CAD build for the part. Positions are in the model's coordinates, mm. A direction names the side the tool comes from. Round coordinates to 2 decimals unless told otherwise and drop trailing zeros. Write each loop counter-clockwise with the first axis right and the second up, starting at its lowest first coordinate (ties: lowest second). Pieces come first, ordered by that corner, then holes. Notation, with made-up numbers: (51.25, 89) -> (85.25, 89) arc R21 cw to (85.25, 102) -> close; hole circle Ø8 at (72.5, 11.25). An arc over 180 degrees is marked (long way). Answer in a Markdown table with one row per item. Add a question column.
```python
from build123d import *

# Parameters (mm, degrees)
SKETCH1_R                       = 60
SKETCH1_R_2                     = 45
BOSS_EXTRUDE1_DEPTH             = 3
CUT_EXTRUDE1_DEPTH              = 85.905830189
CIRPATTERN1_COUNT               = 8
SKETCH3_R                       = 2.1
CUT_EXTRUDE2_DEPTH              = 85.905830189
CIRPATTERN2_COUNT               = 4
SCHNITT_LINEAR_AUSTRAGEN1_DEPTH = 85.905830189
VERRUNDUNG2_R                   = 2
KREISMUSTER7_COUNT              = 4
VERRUNDUNG2_OF_KREISMUSTER7_R   = 2


with BuildPart() as part:
    # Sketch1 → Boss-Extrude1 (new body)
    with BuildSketch(Plane(origin=(0, 0, 0), x_dir=(1, 0, 0), z_dir=(0, 1, 0))):
        with Locations(Location((0, 0, 0), (0, 0, 270))):
            Circle(SKETCH1_R)
        with Locations(Location((0, 0, 0), (0, 0, 270))):
            Circle(SKETCH1_R_2, mode=Mode.SUBTRACT)
    extrude(amount=BOSS_EXTRUDE1_DEPTH)

    # Sketch2 → Cut-Extrude1 (cut, through all)
    with BuildSketch(Plane(origin=(0, 3, 0), x_dir=(1, 0, 0), z_dir=(0, 1, 0))):
        with BuildLine():
            Line((12.399026137, 46.273795509), (12.153476553, 45.357391985))
            ThreePointArc((12.153476553, 45.357391985), (12.332388249, 43.876840862), (13.485952537, 42.931679261))
            Line((13.485952537, 42.931679261), (-13.485952537, 42.931679261))
            ThreePointArc((-13.485952537, 42.931679261), (-12.332388249, 43.876840862), (-12.153476553, 45.357391985))
            Line((-12.153476553, 45.357391985), (-12.399026137, 46.273795509))
            ThreePointArc((-12.399026137, 46.273795509), (-12.051156799, 48.63074892), (-10.0950767, 49.990893435))
            ThreePointArc((-10.0950767, 49.990893435), (0, 51), (10.0950767, 49.990893435))
            ThreePointArc((10.0950767, 49.990893435), (12.051156799, 48.63074892), (12.399026137, 46.273795509))
        make_face()
    cut_extrude1 = extrude(amount=-CUT_EXTRUDE1_DEPTH, mode=Mode.SUBTRACT)

    # CirPattern1: Cut-Extrude1 ×8 about axis
    cirpattern1_axis = Axis((0, 0, 0), (0, 1, 0))
    for i in range(1, CIRPATTERN1_COUNT):
        add(cut_extrude1.rotate(cirpattern1_axis, i * 360 / CIRPATTERN1_COUNT), mode=Mode.SUBTRACT)

    # Sketch3 → Cut-Extrude2 (cut, through all)
    with BuildSketch(Plane(origin=(0, 3, 0), x_dir=(1, 0, 0), z_dir=(0, 1, 0))):
        with Locations(Location((38.890872965, 38.890872965, 0), (0, 0, 270))):
            Circle(SKETCH3_R)
    cut_extrude2 = extrude(amount=-CUT_EXTRUDE2_DEPTH, mode=Mode.SUBTRACT)

    # CirPattern2: Cut-Extrude2 ×4 about axis
    cirpattern2_axis = Axis((0, 0, 0), (0, 1, 0))
    for i in range(1, CIRPATTERN2_COUNT):
        add(cut_extrude2.rotate(cirpattern2_axis, i * 360 / CIRPATTERN2_COUNT), mode=Mode.SUBTRACT)

    # Skizze1 → Schnitt-Linear austragen1 (cut, through all)
    with BuildSketch(Plane(origin=(0, 3, 0), x_dir=(1, 0, 0), z_dir=(0, 1, 0))):
        with BuildLine():
            Line((-12.986376836, 58.577760427), (-12.120618381, 54.672576399))
            ThreePointArc((-12.120618381, 54.672576399), (0, 56), (12.120618381, 54.672576399))
            Line((12.120618381, 54.672576399), (12.986376836, 58.577760427))
            ThreePointArc((12.986376836, 58.577760427), (0, 60), (-12.986376836, 58.577760427))
        make_face()
    schnitt_linear_austragen1 = extrude(amount=-SCHNITT_LINEAR_AUSTRAGEN1_DEPTH, mode=Mode.SUBTRACT)

    # Verrundung2
    verrundung2_edges = [part.edges().sort_by_distance(p)[0] for p in [
        (-12.986376836, 1.5, -58.577760427),
        (-12.120618381, 1.5, -54.672576399),
        (12.986376836, 1.5, -58.577760427),
        (12.120618381, 1.5, -54.672576399),
    ]]
    fillet(verrundung2_edges, radius=VERRUNDUNG2_R - 0.0001)  # a hair under: the kernel refuses the full size

    # Kreismuster7: Schnitt-Linear austragen1 ×4 about axis
    kreismuster7_axis = Axis((0, 0, 0), (0, 1, 0))
    for i in range(1, KREISMUSTER7_COUNT):
        add(schnitt_linear_austragen1.rotate(kreismuster7_axis, i * 360 / KREISMUSTER7_COUNT), mode=Mode.SUBTRACT)

    # Verrundung2 of Kreismuster7
    verrundung2_of_kreismuster7_edges = [part.edges().sort_by_distance(p)[0] for p in [
        (-58.577760427, 1.5, 12.986376836),
        (-54.672576399, 1.5, 12.120618381),
        (-58.577760427, 1.5, -12.986376836),
        (-54.672576399, 1.5, -12.120618381),
        (12.986376836, 1.5, 58.577760427),
        (12.120618381, 1.5, 54.672576399),
        (-12.986376836, 1.5, 58.577760427),
        (-12.120618381, 1.5, 54.672576399),
        (58.577760427, 1.5, -12.986376836),
        (54.672576399, 1.5, -12.120618381),
        (58.577760427, 1.5, 12.986376836),
        (54.672576399, 1.5, 12.120618381),
    ]]
    fillet(verrundung2_of_kreismuster7_edges, radius=VERRUNDUNG2_OF_KREISMUSTER7_R - 0.0001)  # a hair under: the kernel refuses the full size


solid = part.part
```
Item 1: Two-plate mould, pull along X, no slides. Class faces 1 (the cylindrical face through (51, 2, 0)), 2 (the flat face through (43.4, 3, -13.2)), 3 (the cylindrical face through (-56, 2, 0)): +X half, -X half, draft (parallel to the pull), parting line (faces both ways), or undercut.
Item 2: Saw through at C-C on y = 1.8. Count the separate pieces of the cut face and the enclosed holes in it, then the cut area to 3 significant figures.
Item 3: Tool access for faces 4 (the cylindrical face through (0, 2, -56)), 5 (the cylindrical face through (-17.272, 1.479, 41.553)): list every direction of +Z, -Z, +X, -X, +Y, -Y with a clear straight run to the whole face (end or side of a thin tool).
Item 4: Pin check, flat tips, straight feed: pin 1 (1.5 mm diameter, centred on y = 1, z = -13.5, fed in from +X); pin 2 (5 mm diameter, centred on x = -38.89, z = 38.89, fed in from +Y). Stop position of each tip, or through.
Item 5: Drill centre lines: probe 1 along Z at (x, y) = (-41.5, 0.45); probe 2 along Z at (x, y) = (45, 1.6); probe 3 along Z at (x, y) = (-38, 2.4). Where is each one in solid material? Low to high.
Item 6: Saw through at B-B on z = 17.5. Give the cut face in (x, y).
Item 7: Saw through at A-A on x = 32. Give the cut face in (y, z), then the cut area to 3 significant figures.
Recorded:
| question | item | result |
|---|---|---|
| 1 | face 1 | undercut |
| 1 | face 2 | draft |
| 1 | face 3 | -X half |
| 2 | separate pieces | 1 |
| 2 | enclosed holes | 5 |
| 2 | area | 3,300 mm2 |
| 3 | face 4 | -Z, +Y, -Y |
| 3 | face 5 | +Y, -Y |
| 4 | pin 1 | x = 58.14 |
| 4 | pin 2 | y = 3 |
| 5 | probe 1 | -43.33 to -29.64, -23.96 to -17.4, 17.4 to 23.96, 29.64 to 43.33 |
| 5 | probe 2 | -39.69 to -12.09, 12.09 to 39.69 |
| 5 | probe 3 | -46.43 to -40.79, -36.99 to -34.01, 34.01 to 36.99, 40.79 to 46.43 |
| 6 | outline | (-57.39, 0) -> (-41.46, 0) -> (-41.46, 3) -> (-57.39, 3) -> close; (41.46, 0) -> (57.39, 0) -> (57.39, 3) -> (41.46, 3) -> close |
| 7 | outline | (0, -50.75) -> (3, -50.75) -> (3, -39.71) -> (0, -39.71) -> close; (0, 39.71) -> (3, 39.71) -> (3, 50.75) -> (0, 50.75) -> close |
| 7 | area | 66.3 mm2 |
